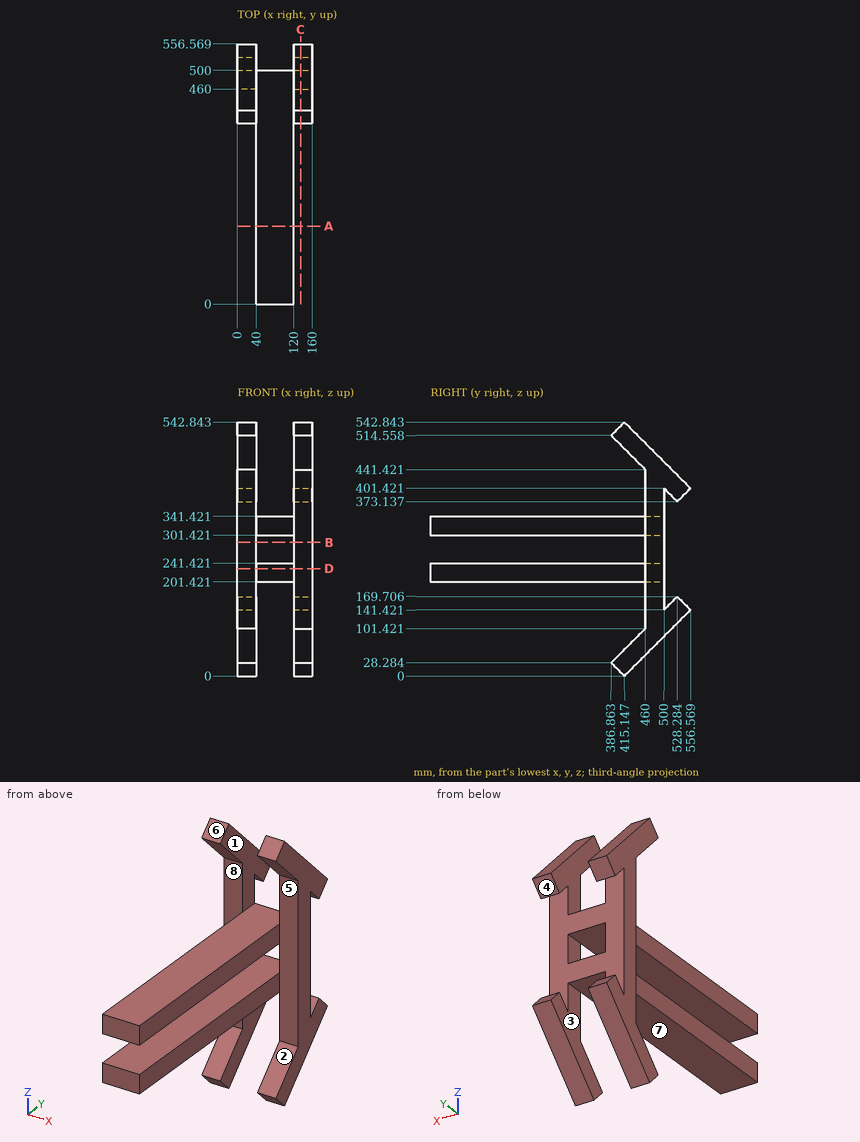
Verification items for this drawing (mm, ordinates from the low corner). A direction names the side the tool comes from. Coordinates: 2 decimals unless noted, no trailing zeros. Write each loop counter-clockwise with the first axis right and the second up, starting at its lowest first coordinate (ties: lowest second). Pieces come first, ordered by that corner, then holes. Notation, with made-up numbers: M 28,56 L 45,56 A12 cw 45,72 Z; hole C 57,31 d8. An arc over 180 degrees is marked long. Answer as a JSON object with one key per item and string values. Group by question number.
(1) Gauge pin test, flat ends, axial feed: pin 1 (12 mm diameter, centred on x = 11.5, z = 255, fed in from -Y); pin 2 (2 mm diameter, centred on x = 136, z = 414, fed in from +Y); pin 3 (4 mm diameter, centred on x = 68, y = 173, fed in from +Z). Record the tip position at first contact, or that the pin passes through.
(2) Cross-section at C-C, the plane x = 135. Record the cut outline in (y, z) (1 decimal).
(3) Material ranges on line 1 (Z direction, x = 67.5, y = 199); line 2 (Y direction, x = 47, z = 215); line 3 (Z direction, x = 18.5, y = 454) (1 decimal), recorded low to high.
(4) Cross-section at D-D, the plane z = 229.5. Record the cut outline in (x, y), and give its area (3 significant figures).
(5) Tool access check on the marked faces 1, 2, 3 and 4. Record the directions out of +Z, -Z, +X, -X, +Y, -Y that give a thin tool (end or side, any length) a straight path to the whole face; none if there is none.
(6) Release check for a two-part mould opening along Z. For the marked faces 5, 6, 7 and 8 record: +Z half, -Z half, draft (parallel to the pull), parting line (faces both ways), or undercut.
(7) Cross-section at B-B, the plane z = 286. Record the cut outline in (x, y).
(8) Cross-section at A-A, the plane y = 167. Record the cut outline in (x, z).
Reply:
{
 "1": {"pin 1": "y = 460", "pin 2": "y = 544.99", "pin 3": "z = 341.42"},
 "2": {"outline": "M 386.9,28.3 L 415.1,0 L 556.6,141.4 L 528.3,169.7 L 500,141.4 L 500,401.4 L 528.3,373.1 L 556.6,401.4 L 415.1,542.8 L 386.9,514.6 L 460,441.4 L 460,101.4 Z"},
 "3": {"line 1": "201.42 to 241.42, 301.42 to 341.42", "line 2": "0 to 500", "line 3": "38.9 to 95.4, 447.4 to 504"},
 "4": {"outline": "M 0,460 L 40,460 L 40,0 L 120,0 L 120,460 L 160,460 L 160,500 L 0,500 Z", "area": "43,200 mm²"},
 "5": {"face 1": "+Z, +Y, -Y", "face 2": "+X, -X, -Y", "face 3": "-Z, +Y, -Y", "face 4": "+X, -X, +Y"},
 "6": {"face 5": "undercut", "face 6": "+Z half", "face 7": "-Z half", "face 8": "undercut"},
 "7": {"outline": "M 0,460 L 40,460 L 40,500 L 0,500 Z; M 120,460 L 160,460 L 160,500 L 120,500 Z"},
 "8": {"outline": "M 40,201.42 L 120,201.42 L 120,241.42 L 40,241.42 Z; M 40,301.42 L 120,301.42 L 120,341.42 L 40,341.42 Z"}
}
